```python
from build123d import *

# Parameters (mm, degrees)
F1_DEPTH = 2
F2_R     = 5
F3_R     = 2.5
F4_DEPTH = 3


with BuildPart() as f1:
    # F0 (on Front) → F1 (new body)
    with BuildSketch(Plane.XZ):
        Polygon((45, 12.5), (-12.5, 12.5), (-12.5, -45), (0, -45), (0, 0), (45, 0), align=None)
    extrude(amount=F1_DEPTH)

    # F2
    f2_edges = [f1.edges().sort_by_distance(p)[0] for p in [
        (-12.5, -1, 12.5),
        (0, -1, 0),
    ]]
    fillet(f2_edges, radius=F2_R)

    # F3 (on Front) → F4 (join)
    with BuildSketch(Plane.XZ):
        with Locations((24.5, 5.5)):
            Circle(F3_R)
        with Locations((-5.5, -24.5)):
            Circle(F3_R)
    extrude(amount=-F4_DEPTH)


solid = f1.part
```
The model under review builds one solid part; all positions refer to its coordinate system, in mm. A direction names the side the tool comes from. Give positions to 0.01 mm unless a question says otherwise; leave off trailing zeros. Write each loop counter-clockwise with the first axis right and the second up, starting at its lowest first coordinate (ties: lowest second). Pieces come first, ordered by that corner, then holes. Notation, with made-up numbers: (27.5, 81.25) - (54.5, 81.25) arc R25 cw to (54.5, 109.25) - close; hole circle Ø2 at (-13.75, -35). An arc over 180 degrees is marked (long way). Answer in a Markdown table with one row per item. Add a question column.
1. We need section A-A on z = -24.5. Write out the cut boundary in (x, y).
2. Insertion check: P1, Ø1.5, axis at x = -4, y = 1, coming from the -Z side; P2, Ø8, axis at x = 1, z = -14, coming from the +Y side; P3, Ø0.6, axis at x = 28, y = -0.5, coming from the -Z side. Each pin has a flat end and moves straight along its axis. Give the tip position at first contact, or say it passes through.
3. Wall thickness on line 1 along X through (y, z) = (-1.3, -40); line 2 along Y through (x, z) = (-1, -3.5); line 3 along Z through (x, y) = (30.5, -1.7): over which ranges is each line inside the solid? List them lowest first. Write a range as [from, to].
4. We need section C-C on x = 24.5. Write out the cut boundary in (y, z), then the cut area to 3 significant figures.
5. We need section D-D on x = 11. Write out the cut boundary in (y, z), then the cut area to 3 significant figures.
6. Tool access review of faces 1 (the flat face through (0, -1, -25)), 2 (the flat face through (24, 3, 6)), 3 (the cylindrical face through (22.66, 1.48, 7.19)): name each direction out of +Z, -Z, +X, -X, +Y, -Y from which nothing blocks a thin tool from reaching the whole face with its end or side.
7. We need section B-B on y = 2. Write out the cut boundary in (x, z).
Ans:
| question | item | result |
|---|---|---|
| 1 | outline | (-12.5, -2) - (0, -2) - (0, 0) - (-3, 0) - (-3, 3) - (-8, 3) - (-8, 0) - (-12.5, 0) - close |
| 2 | P1 | stops at z = -26.88 |
| 2 | P2 | stops at y = 0 |
| 2 | P3 | stops at z = 0 |
| 3 | line 1 | x = [-12.5, 0] |
| 3 | line 2 | y = [-2, 0] |
| 3 | line 3 | z = [0, 12.5] |
| 4 | outline | (-2, 0) - (0, 0) - (0, 3) - (3, 3) - (3, 8) - (0, 8) - (0, 12.5) - (-2, 12.5) - close |
| 4 | area | 40.0 mm^2 |
| 5 | outline | (-2, 0) - (0, 0) - (0, 12.5) - (-2, 12.5) - close |
| 5 | area | 25.0 mm^2 |
| 6 | face 1 | -Z, +X, +Y, -Y |
| 6 | face 2 | +Z, -Z, +X, -X, +Y |
| 6 | face 3 | +Y |
| 7 | outline | circle Ø5 at (-5.5, -24.5); circle Ø5 at (24.5, 5.5) |
